Source: CAD feature listing. Evaluate the final solid. Frame: model axes, mm. A direction names the side the tool comes from. Give positions to 0.01 mm unless a question says otherwise; leave off trailing zeros. Loops run counter-clockwise (first coordinate to the right, second up) from the corner with the lowest first, then second, coordinate; pieces in that order, holes last.
Solid Edge part; units mm, degrees
sketch "Sketch1" plane through (0, 0, 0) normal (0, 0, 1) x (1, 0, 0)
  arc A0 (-12.5347, 17.468) -> (12.5347, 17.468) centre (0, 0) cw
  arc A1 (17.468, 12.5347) -> (17.468, -12.5347) centre (0, 0) cw
  arc A2 (12.5347, -17.468) -> (-12.5347, -17.468) centre (0, 0) cw
  arc A3 (-17.468, -12.5347) -> (-17.468, 12.5347) centre (0, 0) cw
  arc A4 (-12.5347, 17.468) -> (-17.468, 12.5347) centre (-15.2028, 15.2028) cw
  arc A5 (17.468, 12.5347) -> (12.5347, 17.468) centre (15.2028, 15.2028) cw
  arc A6 (12.5347, -17.468) -> (17.468, -12.5347) centre (15.2028, -15.2028) cw
  arc A7 (-17.468, -12.5347) -> (-12.5347, -17.468) centre (-15.2028, -15.2028) cw
extrude "Protrusion1" add sketch "Sketch1" against normal blind 5
sketch "Sketch2" plane through (0, 0, 0) normal (0, 0, 1) x (1, 0, 0)
  circle A0 centre (-17.5, 0) radius 1.75
  circle A1 centre (17.5, 0) radius 1.75
extrude "Cutout1" cut sketch "Sketch2" against normal through all
sketch "Sketch3" plane through (0, 0, 0) normal (0, 0, 1) x (1, 0, 0)
  circle A0 centre (-17.5, 0) radius 3
  circle A1 centre (17.5, 0) radius 3
extrude "VaciadoExtruido_2" cut sketch "Sketch3" against normal blind 4
chamfer "Chaflán_1" distance 0.4 angle 45 20 edges at (-20.5, 0, 0) (14.5, 0, 0) (-12.7279, -12.7279, 0) (0, -21.5, 0) (12.7279, -12.7279, 0) (21.5, 0, 0) (12.7279, 12.7279, 0) (0, 21.5, 0) (-12.7279, 12.7279, 0) (-21.5, 0, 0) (15.75, 0, -5) (-19.25, 0, -5) (-12.7279, -12.7279, -5) (-21.5, 0, -5) (-12.7279, 12.7279, -5) (0, 21.5, -5) (12.7279, 12.7279, -5) (21.5, 0, -5) (12.7279, -12.7279, -5) (0, -21.5, -5)
sketch "Sketch4" plane through (0, 0, 0) normal (0, 0, 1) x (0, 1, 0)
  line L0 (-5.25, 5.75) -> (5.25, 5.75)
  line L1 (5.25, 5.75) -> (5.25, 0.25)
  line L2 (5.25, 0.25) -> (-5.25, 0.25)
  line L3 (-5.25, 0.25) -> (-5.25, 5.75)
  line L4 (-5.25, -5.75) -> (-5.25, -0.25)
  line L5 (-5.25, -0.25) -> (5.25, -0.25)
  line L6 (5.25, -0.25) -> (5.25, -5.75)
  line L7 (5.25, -5.75) -> (-5.25, -5.75)
extrude "Cutout2" cut sketch "Sketch4" against normal through all
fillet "Redondeo_1" radius 2 4 edges at (-5.75, 5.25, -2.5) (-0.25, 5.25, -2.5) (0.25, 5.25, -2.5) (5.75, 5.25, -2.5)
1) Contact query for flat-ended pins moving along their axis: P1, Ø2.5, axis at y = -2.5, z = -3, coming from the -X side; P2, Ø1.8, axis at x = 17.5, y = 1, coming from the +Z side; P3, Ø1.6, axis at x = 3, z = -3.5, coming from the -Y side; P4, Ø2, axis at x = -17.5, y = 0, coming from the -Z side. Output: stop coordinate, or through.
Checks:
P1: stops at x = -21.46
P2: stops at z = -4
P3: stops at y = -21.39
P4: passes through
2) Pull-direction query (Y, two-part tool) for faces 1 (the conical face through (-0.18, 21.21, -0.11)), 2 (the flat face through (3, -5.25, -2)), 3 (the conical face through (-21.21, 0.18, -4.89)), 4 (the flat face through (0, 5, -5)); classes: released by +Y, released by -Y, zero draft, split by the parting line, or undercut.
Checks:
face 1: released by +Y
face 2: undercut
face 3: split by the parting line
face 4: zero draft
3) Ray query, probe 1 along Y at (x, z) = (-17, -2.55); probe 2 along X at (y, z) = (1.5, -2.4); probe 3 along Y at (x, z) = (-17.5, -4.4). Return the intervals inside material, ascending.
Checks:
probe 1: y = -12.2 to -2.96, 2.96 to 12.2
probe 2: x = -21.45 to -20.1, -14.9 to -5.75, -0.25 to 0.25, 5.75 to 14.9, 20.1 to 21.45
probe 3: y = -12.49 to -1.75, 1.75 to 12.49
4) Cut plane B-B (y = 0). State how many separate pieces and enclosed holes the cut face has, and give its area (3 significant figures).
Checks:
separate pieces: 5
enclosed holes: 0
area: 104 mm2
5) Cut plane A-A (z = -1.65). Return loops of the section in (x, y).
Checks:
outline: (-17.47, -12.53) arc R3.5 cw to (-12.53, -17.47) arc R21.5 ccw to (12.53, -17.47) arc R3.5 cw to (17.47, -12.53) arc R21.5 ccw to (17.47, 12.53) arc R3.5 cw to (12.53, 17.47) arc R21.5 ccw to (-12.53, 17.47) arc R3.5 cw to (-17.47, 12.53) arc R21.5 ccw to start; hole circle Ø6 at (-17.5, 0); hole (-5.75, -5.25) - (-0.25, -5.25) - (-0.25, 3.25) arc R2 ccw to (-2.25, 5.25) - (-3.75, 5.25) arc R2 ccw to (-5.75, 3.25) - close; hole (0.25, -5.25) - (5.75, -5.25) - (5.75, 3.25) arc R2 ccw to (3.75, 5.25) - (2.25, 5.25) arc R2 ccw to (0.25, 3.25) - close; hole circle Ø6 at (17.5, 0)
6) Reachability of faces 5 (the flat face through (-0.25, -1, -2)), 6 (the cylindrical face through (-20.5, 0.1, -2.2)), 7 (the conical face through (0.18, -21.21, -0.11)) from +Z, -Z, +X, -X, +Y, -Y: full face, straight path, thin tool, end or side. Return the list, or none.
Checks:
face 5: +Z, -Z
face 6: +Z
face 7: +Z, -Y
